The figure shows three views and two pictorial views of one solid part (mm, origin at its lowest corner). Answer the questions. A direction names the side the tool comes from. Round coordinates to 2 decimals unless told otherwise and drop trailing zeros. Write each loop counter-clockwise with the first axis right and the second up, starting at its lowest first coordinate (ties: lowest second). Pieces come first, ordered by that corner, then holes.
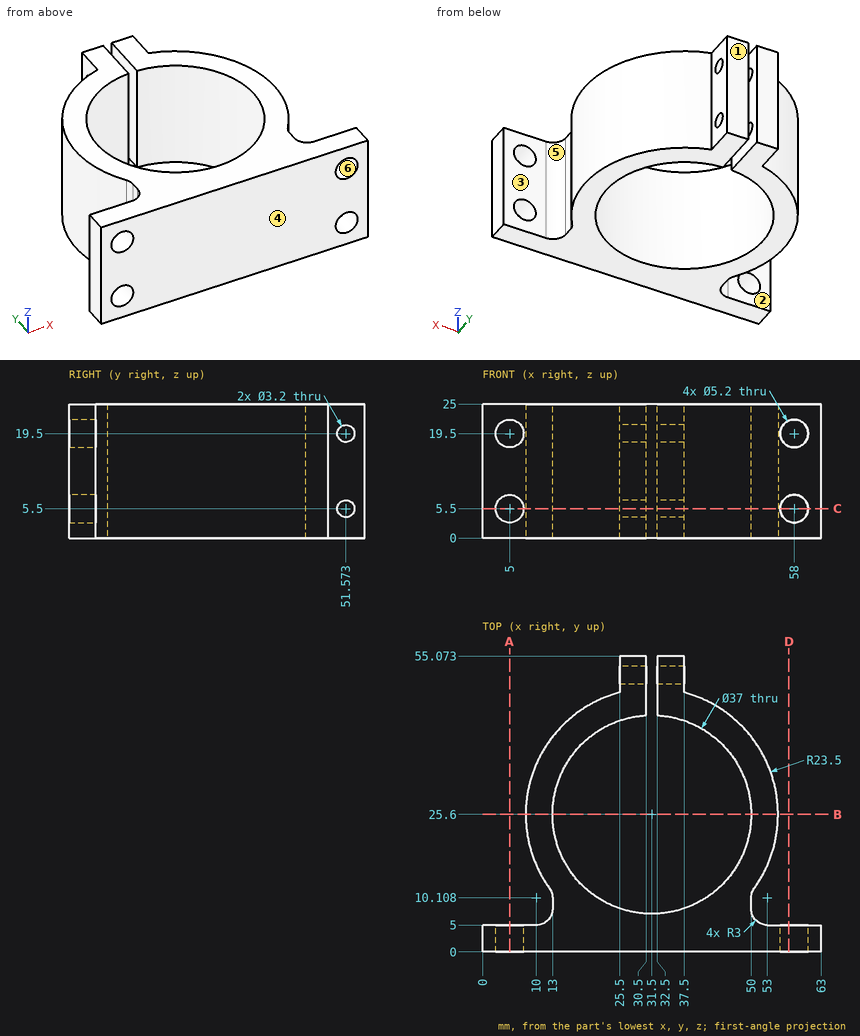
Q1. Section B-B (y = 25.6) is taken. Determine the outline of the cut face in (x, z).
Verdict:
outline: (8, 0) - (13, 0) - (13, 25) - (8, 25) - close; (50, 0) - (55, 0) - (55, 25) - (50, 25) - close
Q2. Determine the mould class of the marked faces 4, 5 and 6 for opening direction Y: pulls with the +Y half, pulls with the -Y half, needs draft (parallel to the pull), parting line crosses it, or undercut.
Verdict:
face 4: pulls with the -Y half
face 5: undercut
face 6: needs draft
Q3. Section D-D (x = 57) is taken. Determine the outline of the cut face in (y, z), then the cut area to 3 significant figures.
Verdict:
outline: (0, 0) - (5, 0) - (5, 3.1) - (0, 3.1) - close; (0, 7.9) - (5, 7.9) - (5, 17.1) - (0, 17.1) - close; (0, 21.9) - (5, 21.9) - (5, 25) - (0, 25) - close
area: 77.0 mm2
Q4. Which of the six approach directions +Z, -Z, +X, -X, +Y, -Y give full straight-line access (tool end or side, diameter ignored) to the marked faces 1, 2 and 3?
Verdict:
face 1: +Z, -Z, +X, -X, +Y
face 2: +Z, -Z, -X
face 3: +Z, -Z, +X
Q5. Section C-C (z = 5.5) is taken. State how many separate pieces and enclosed holes the cut face has, then the cut area to 3 significant figures.
Verdict:
separate pieces: 5
enclosed holes: 0
area: 941 mm2
Q6. Flat-ended cylindrical pins translate along their axes: pin 1 Ø1.5 at (y, z) = (13, 12) entering from +X; pin 2 Ø1.5 at (y, z) = (34, 12.5) entering from +X; pin 3 Ø4 at (y, z) = (35.5, 17) entering from +X. Find the tip coordinate at first contact, or state that the pin passes through.
Verdict:
pin 1: stops at x = 51.79
pin 2: stops at x = 53.72
pin 3: stops at x = 53.63
Q7. Section A-A (x = 5) is taken. Determine the outline of the cut face in (y, z), then the cut area to 3 significant figures.
Verdict:
outline: (0, 0) - (5, 0) - (5, 2.9) - (0, 2.9) - close; (0, 8.1) - (5, 8.1) - (5, 16.9) - (0, 16.9) - close; (0, 22.1) - (5, 22.1) - (5, 25) - (0, 25) - close
area: 73.0 mm2
Q8. Straight lines are drawn through the part: probe 1 along Z at (x, y) = (58, 2); probe 2 along X at (y, z) = (2.35, 19.5); probe 3 along X at (y, z) = (49, 11.75). For each, find the intervals that lie inside material, in ascending order.
Verdict:
probe 1: z = 0 to 2.9, 8.1 to 16.9, 22.1 to 25
probe 2: x = 0 to 2.4, 7.6 to 55.4, 60.6 to 63
probe 3: x = 25.5 to 30.5, 32.5 to 37.5
